Source: CAD feature listing. Evaluate the final solid. Frame: model axes, mm. Face numbers are marked on the shaded views. A direction names the side the tool comes from. Round coordinates to 2 decimals unless told otherwise and drop trailing zeros. Loops run counter-clockwise (first coordinate to the right, second up) from the corner with the lowest first, then second, coordinate; pieces in that order, holes last. Notation, with made-up numbers: (-17.75, -33.5) -> (34.25, -33.5) arc R6 cw to (34.25, -28.5) -> close; hole circle Ø9 at (67.25, 51). An arc over 180 degrees is marked (long way). Put each result on its own line as item: value. Start each with the question number.
1. Draft query along X for the marked faces 1, 2 and 3. Return one class per face: pulls with the +X half, pulls with the -X half, needs draft (parallel to the pull), parting line crosses it, or undercut.
2. Cut plane A-A (z = -15.25). Return the cut outline in (x, y).
3. Cut plane D-D (y = 20). Return the cut outline in (x, z), then the cut area to 3 significant figures.
4. Cut plane C-C (z = -24.5). State how many separate pieces and enclosed holes the cut face has, then the cut area to 3 significant figures.
5. Set-up query: the marked faces 4, 5 and 6. Return all of +Z, -Z, +X, -X, +Y, -Y with unobstructed straight access to the full face (end or side cutting, diameter ignored); none if empty.
6. Contact query for flat-ended pins moving along their axis: pin 1 (10 mm diameter, centred on x = -13, z = -26, fed in from +Y); pin 2 (3.5 mm diameter, centred on y = 20, z = -23, fed in from -X); pin 3 (3 mm diameter, centred on x = 0, y = -9, fed in from +Z). Output: stop coordinate, or through.
7. Material intervals for L1, parallel to Y at x = 18, z = -20.5; L2, parallel to X at y = -12.2, z = -23; L3, parallel to X at y = 13, z = -29.25, sorted ascending.
8. Cut plane B-B (x = -15). Return the cut outline in (y, z), then the cut area to 3 significant figures.
```python
from build123d import *

# Parameters (mm, degrees)
SKETCH005_W             = 58
SKETCH005_H             = 20
SKETCH005_R             = 2.75
PAD004_DEPTH            = 8
SKETCH006_R             = 2.25
PAD005_DEPTH            = 4
POCKET005_DEPTH         = 4
SKETCH011_W             = 15
SKETCH011_H             = 2.666667
POCKET007_DEPTH         = 20
SKETCH012_W             = 18
SKETCH012_H             = 3
POCKET008_DEPTH         = 8
FILLET_R                = 0.5
BODY002_PLACEMENT_ANGLE = 180


with BuildPart() as part:
    # Sketch005 → Pad004 (new body)
    with BuildSketch(Plane.XZ):
        Rectangle(SKETCH005_W, SKETCH005_H)
        Circle(SKETCH005_R, mode=Mode.SUBTRACT)
    extrude(amount=PAD004_DEPTH)

    # Sketch006 (on Face4 of Pad004) → Pad005 (join)
    with BuildSketch(Plane(origin=(-29, 0, 0), x_dir=(0, 0, -1), z_dir=(-1, 0, 0))):
        with BuildLine():
            Line((-10, 0), (10, 0))
            Line((10, 0), (10, 30.5))
            ThreePointArc((10, 30.5), (0, 40.5), (-10, 30.5))
            Line((-10, 30.5), (-10, 0))
        make_face()
        with Locations((0, 35)):
            Circle(SKETCH006_R, mode=Mode.SUBTRACT)
    pad005 = extrude(amount=PAD005_DEPTH)

    # Mirrored003: Pad005 across YZ
    add(pad005.mirror(Plane.YZ))

    # Sketch007 (on Face5 of Mirrored003) → Pocket005 (cut)
    with BuildSketch(Plane.XZ.offset(8)):
        Polygon((2.374981, 4.113632), (-2.375019, 4.11361), (-4.75, -2.2e-05), (-2.374981, -4.113632), (2.375019, -4.11361), (4.75, 2.2e-05), align=None)
    extrude(amount=-POCKET005_DEPTH, mode=Mode.SUBTRACT)

    # Sketch011 (on Face14 of Pocket005) → Pocket007 (cut)
    with BuildSketch(Plane(origin=(0, 0, 10), x_dir=(-1, 0, 0), z_dir=(0, 0, 1))):
        with Locations((-19.5, 4.169504)):
            Rectangle(SKETCH011_W, SKETCH011_H)
    pocket007 = extrude(amount=-POCKET007_DEPTH, mode=Mode.SUBTRACT)

    # Mirrored004: Pocket007 across YZ
    add(pocket007.mirror(Plane.YZ), mode=Mode.SUBTRACT)

    # Sketch012 (on Face3 of Mirrored004) → Pocket008 (cut)
    with BuildSketch(Plane(origin=(0, 0, 0), x_dir=(1, 0, 0), z_dir=(0, 1, 0))):
        with Locations((0, 8.5)):
            Rectangle(SKETCH012_W, SKETCH012_H)
    extrude(amount=-POCKET008_DEPTH, mode=Mode.SUBTRACT)

    # Fillet
    fillet_edges = [part.edges().sort_by_distance(p)[0] for p in [
        (0, -8, -7),
        (9, -8, -8.5),
        (-9, -8, -8.5),
    ]]
    fillet(fillet_edges, radius=FILLET_R)


with BuildPart() as part_1:
    # Body002 placement: moved
    add(part.part.moved(Location((0, -15, -23))).rotate(Axis((0, -15, -23), (1, 0, 0)), BODY002_PLACEMENT_ANGLE))


solid = part_1.part
```
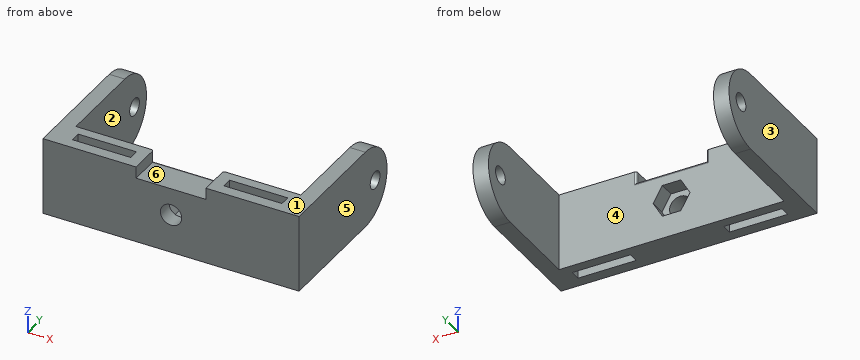
Solution:
1. face 1: needs draft
1. face 2: undercut
1. face 3: pulls with the -X half
2. outline: (-33, -15) -> (-9, -15) -> (-9, -7.5) arc R0.5 ccw to (-9.5, -7) -> (-29, -7) -> (-29, 21.82) -> (-33, 21.82) -> close; (9, -15) -> (33, -15) -> (33, 21.82) -> (29, 21.82) -> (29, -7) -> (9.5, -7) arc R0.5 ccw to (9, -7.5) -> close; hole (-27, -12.16) -> (-12, -12.16) -> (-12, -9.5) -> (-27, -9.5) -> close; hole (12, -12.16) -> (27, -12.16) -> (27, -9.5) -> (12, -9.5) -> close
3. outline: (-33, -31.93) -> (-29, -31.93) -> (-29, -25.25) -> (-33, -25.25) -> close; (-33, -20.75) -> (-29, -20.75) -> (-29, -14.07) -> (-33, -14.07) -> close; (29, -31.93) -> (33, -31.93) -> (33, -25.25) -> (29, -25.25) -> close; (29, -20.75) -> (33, -20.75) -> (33, -14.07) -> (29, -14.07) -> close
3. area: 107 mm^2
4. separate pieces: 4
4. enclosed holes: 2
4. area: 631 mm^2
5. face 4: +Z, -Z, +Y
5. face 5: +Z, -Z, +X, +Y, -Y
5. face 6: +Z, +Y, -Y
6. pin 1: stops at y = -7
6. pin 2: passes through
6. pin 3: stops at z = -16
7. L1: y = -15 to -12.16, -9.5 to -7
7. L2: x = -33 to -2.75, 2.75 to 33
7. L3: x = -33 to -29, 29 to 33
8. outline: (-15, -33) -> (-12.16, -33) -> (-12.16, -13) -> (-15, -13) -> close; (-9.5, -33) -> (-7, -33) -> (-7, -13) -> (-9.5, -13) -> close
8. area: 107 mm^2
